from build123d import *

# Parameters (mm, degrees)
SKETCH2_R           = 1
BOSS_EXTRUDE1_DEPTH = 6
CHAMFER1_SIZE       = 0.3
SKETCH6_W           = 2
SKETCH6_H           = 1.8
CUT_EXTRUDE1_DEPTH  = 1
CHAMFER2_SIZE       = 0.15
CHAMFER3_SIZE       = 0.1


with BuildPart() as part:
    # Sketch2 → Boss-Extrude1 (new body)
    with BuildSketch(Plane(origin=(0, 0, 0), x_dir=(0, 0, -1), z_dir=(1, 0, 0))):
        Circle(SKETCH2_R)
    extrude(amount=-BOSS_EXTRUDE1_DEPTH)

    # Chamfer1
    chamfer1_edges = [part.edges().sort_by_distance(p)[0] for p in [
        (0, 0, 1),
    ]]
    chamfer(chamfer1_edges, length=CHAMFER1_SIZE)

    # Sketch6 → Revolve1 (revolve)
    with BuildSketch(Plane.XY):
        with Locations((-7, 0.9)):
            Rectangle(SKETCH6_W, SKETCH6_H)
    revolve(axis=Axis((-6, 0, 0), (-1, 0, 0)))

    # Sketch7 → Cut-Extrude1 (cut)
    with BuildSketch(Plane.ZY.offset(8)):
        Polygon((0, 0.894892917), (-0.775, 0.447446459), (-0.775, -0.447446459), (0, -0.894892917), (0.775, -0.447446459), (0.775, 0.447446459), align=None)
    extrude(amount=-CUT_EXTRUDE1_DEPTH, mode=Mode.SUBTRACT)

    # Cut-Extrude2 cone 1 section (through the dimple's axis) → Cut-Extrude2 (revolve, cut)
    with BuildSketch(Plane(origin=(-8, 0, 0), x_dir=(0, 0, 1), z_dir=(0, 1, 0))):
        Polygon((0, 0), (0.944892917, 0), (0, 0.944892917), align=None)
    revolve(axis=Axis((-8, 0, 0), (1, 0, 0)), mode=Mode.SUBTRACT)

    # Chamfer2
    chamfer2_edges = [part.edges().sort_by_distance(p)[0] for p in [
        (-8, -1.8, 0),
    ]]
    chamfer(chamfer2_edges, length=CHAMFER2_SIZE)

    # Chamfer3
    chamfer3_edges = [part.edges().sort_by_distance(p)[0] for p in [
        (-6, 0, 1),
    ]]
    chamfer(chamfer3_edges, length=CHAMFER3_SIZE)


solid = part.part
Read the model definition and answer for the solid it produces. Units are mm, in the model's axes. A direction names the side the tool comes from. Give positions to 0.01 mm unless a question says otherwise; leave off trailing zeros. Write each loop counter-clockwise with the first axis right and the second up, starting at its lowest first coordinate (ties: lowest second). Pieces come first, ordered by that corner, then holes. Notation, with made-up numbers: (-13, -34) -> (25, -34) arc R33 cw to (25, 1) -> close; hole circle Ø2 at (-30.75, -31). An arc over 180 degrees is marked (long way). Answer as a JSON object with one key per item and string values. Group by question number.
1) Consider L1, parallel to X at y = 1, z = -0.75; L2, parallel to Z at x = -5.25, y = -0.45; L3, parallel to X at y = -0.2, z = -0.5. Determine where each line is inside the solid, lowest interval first. Write a range as from..to.
2) Find section B-B (x = -5.5). Write down the section's boundary in (y, z).
3) The mould has two halves that part along Y. Classify faces 1 (the flat face through (-7.5, 0, -0.775)), 2 (the cylindrical face through (-6.912, 1.717, -0.541)), 3 (the flat face through (-6, 1, 1)): +Y half, -Y half, draft (parallel to the pull), parting line (faces both ways), or undercut.
4) Find section A-A (y = 0). Write down the section's boundary in (x, z) (3 decimals), and give its area (3 significant figures).
5) This flat-tipped pin is pushed along its axis until it touches: P1, Ø1.5, axis at x = -1.5, y = 0.5, coming from the +Z side. Where does it stop, or does it pass through?
6) A tool of negligible diameter and unlimited length cuts with its end or side. For faces 4 (the cylindrical face through (-3, -1, 0)), 5 (the flat face through (-8, -1, 1)), 6 (the flat face through (-7.5, 0, 0.775)), from which of +Z, -Z, +X, -X, +Y, -Y can it reach the whole face along a straight path? Write none if from no direction.
Values follow:
{
 "1": {"L1": "x = -8..-6", "L2": "z = -0.89..0.89", "L3": "x = -7..0"},
 "2": {"outline": "circle Ø2 at (0, 0)"},
 "3": {"face 1": "undercut", "face 2": "parting line", "face 3": "draft"},
 "4": {"outline": "(-8, -1.65) -> (-7.85, -1.8) -> (-6, -1.8) -> (-6, -1.1) -> (-5.9, -1) -> (-0.3, -1) -> (0, -0.7) -> (0, 0.7) -> (-0.3, 1) -> (-5.9, 1) -> (-6, 1.1) -> (-6, 1.8) -> (-7.85, 1.8) -> (-8, 1.65) -> (-8, 0.945) -> (-7.83, 0.775) -> (-7, 0.775) -> (-7, -0.775) -> (-7.83, -0.775) -> (-8, -0.945) -> close", "area": "17.5 mm2"},
 "5": {"P1": "stops at z = 1"},
 "6": {"face 4": "+X", "face 5": "+Z, -Z, -X, +Y, -Y", "face 6": "-X"}
}
